from build123d import *

# Parameters (mm, degrees)
F0_W      = 127
F0_H      = 127
F2_DEPTH  = 5.08
F3_W      = 50.8
F3_H      = 58.42
F4_DEPTH  = 5.08
F5_W      = 50.8
F5_H      = 12.7
F6_DEPTH  = 2.54
F7_R      = 5.07999
F9_W      = 120.65
F9_H      = 120.65
F10_DEPTH = 3.175
F11_R     = 4.064
F12_DEPTH = 25.4


# Not quite as in the source:
# - a fillet or chamfer is up to 0.001 mm smaller than in the source, because OpenCascade refuses the exact size


with BuildPart() as f2:
    # F0 (on Top) → F2 (new body)
    with BuildSketch(Plane.XY):
        with Locations((-1.9660266274, -3.4333672374)):
            Rectangle(F0_W, F0_H)
    extrude(amount=-F2_DEPTH)

    # F3 (on face) → F4 (join)
    with BuildSketch(Plane.XY):
        with Locations((0, -96.1433672374)):
            Rectangle(F3_W, F3_H)
    extrude(amount=-F4_DEPTH)

    # F5 (on face) → F6 (cut)
    with BuildSketch(Plane.XZ.offset(125.3533672374)):
        with Locations((0, -11.43)):
            Rectangle(F5_W, F5_H)
    extrude(amount=-F6_DEPTH, mode=Mode.SUBTRACT)

    # F7 (radius 5.08 in the source; OpenCascade refuses exactly that, so slightly less here)
    f7_edges = [f2.edges().sort_by_distance(p)[0] for p in [
        (0, -125.353367, 0),
    ]]
    fillet(f7_edges, radius=F7_R)

    # F9 (on Top) → F10 (cut)
    with BuildSketch(Plane.XY):
        with Locations((-2.4150442332, -3.342743357)):
            Rectangle(F9_W, F9_H)
    extrude(amount=-F10_DEPTH, mode=Mode.SUBTRACT)

    # F11 (on face) → F12 (cut)
    with BuildSketch(Plane.XY):
        with Locations((0, -96.6428003655)):
            Circle(F11_R)
    extrude(amount=-F12_DEPTH, mode=Mode.SUBTRACT)


solid = f2.part
Design review of the part built by this model. Coordinates are the model's own, in mm. A direction names the side the tool comes from. Round coordinates to 2 decimals unless told otherwise and drop trailing zeros. Write each loop counter-clockwise with the first axis right and the second up, starting at its lowest first coordinate (ties: lowest second). Pieces come first, ordered by that corner, then holes. Notation, with made-up numbers: (84.25, 61) -> (102.25, 61) arc R24 cw to (102.25, 93) -> close; hole circle Ø5 at (36, 29). An arc over 180 degrees is marked (long way). One line per item, written item: value. Start each with the question number.
Q1. The part is to be moulded in two halves that separate along X. For faces 1 (the face through (-0.88, -100.61, -2.5)), 2 (the face through (-65.466, -4, -3)), 3 (the face through (-2, -70, 0)), say which applies: pulls with the +X half, pulls with the -X half, needs draft (parallel to the pull), parting line crosses it, or undercut.
Q2. Add section C-C (z = -1.9). Give the boundary of the cut face in (x, y), then the cut area to 3 significant figures.
Q3. Add section B-B (y = 43). Give the boundary of the cut face in (x, z) (3 decimals), then the cut area to 3 significant figures.
Q4. To check wall thickness, follow probe 1 along X at (y, z) = (48, -1.45); probe 2 along Y at (x, z) = (-39, -2.65); probe 3 along Y at (x, z) = (2, -2.65) (3 decimals). State the ranges of each line that lie inside material, in increasing order.
Q5. Insertion check: P1, Ø2, axis at x = -18, z = -1.5, coming from the -Y side; P2, Ø1.6, axis at x = -15.5, z = -2.5, coming from the -Y side; P3, Ø1, axis at x = 1, y = 4.5, coming from the +Z side (3 decimals). Each pin has a flat end and moves straight along its axis. Give the tip position at first contact, or say it passes through.
Q6. Tool access review of faces 4 (the face through (43, -66.933, -3)), 5 (the face through (-3, -2, -3.175)), 6 (the face through (-46, -66.933, -3)): name each direction out of +Z, -Z, +X, -X, +Y, -Y from which nothing blocks a thin tool from reaching the whole face with its end or side.
Q7. Add section D-D (x = -57). Give the boundary of the cut face in (y, z) (3 decimals), then the cut area to 3 significant figures.
Response:
1. face 1: undercut
1. face 2: pulls with the -X half
1. face 3: needs draft
2. outline: (-65.47, -66.93) -> (-25.4, -66.93) -> (-25.4, -124.23) -> (25.4, -124.23) -> (25.4, -66.93) -> (61.53, -66.93) -> (61.53, 60.07) -> (-65.47, 60.07) -> close; hole (-62.74, -63.67) -> (57.91, -63.67) -> (57.91, 56.98) -> (-62.74, 56.98) -> close; hole circle Ø8.13 at (0, -96.64)
2. area: 4,430 mm^2
3. outline: (-65.466, -5.08) -> (61.534, -5.08) -> (61.534, 0) -> (57.91, 0) -> (57.91, -3.175) -> (-62.74, -3.175) -> (-62.74, 0) -> (-65.466, 0) -> close
3. area: 262 mm^2
4. probe 1: x = -65.47 to -62.74, 57.91 to 61.53
4. probe 2: y = -66.93 to -63.67, 56.98 to 60.07
4. probe 3: y = -124.734 to -100.181, -93.105 to -63.668, 56.982 to 60.067
5. P1: stops at y = -124.65
5. P2: stops at y = -125.03
5. P3: stops at z = -3.175
6. face 4: +Z, -Z, +X, -Y
6. face 5: +Z
6. face 6: +Z, -Z, -X, -Y
7. outline: (-66.933, -5.08) -> (60.067, -5.08) -> (60.067, 0) -> (56.982, 0) -> (56.982, -3.175) -> (-63.668, -3.175) -> (-63.668, 0) -> (-66.933, 0) -> close
7. area: 262 mm^2
